from build123d import *
from build123d.topology import SkipClean

# Parameters (mm, degrees)
ESQUISSE1_R             = 2.1
ESQUISSE1_R_2           = 13.5
BOSS_EXTRU_1_DEPTH      = 3
ESQUISSE2_R             = 2.1
ENL_V_MAT_EXTRU_1_DEPTH = 3
ESQUISSE3_R             = 4.1
ESQUISSE3_R_2           = 2.1
BOSS_EXTRU_2_DEPTH      = 2
ENL_V_MAT_EXTRU_2_DEPTH = 3
CONG_1_R                = 20


with BuildPart() as part:
    # Esquisse1 → Boss.-Extru.1 (new body)
    with BuildSketch(Plane.XY):
        Polygon((22.273863607, -59.043416229), (-59.043416229, 22.273863607), (-22.273863607, 59.043416229), (59.043416229, -22.273863607), align=None)
        with Locations((0, 20)):
            Circle(ESQUISSE1_R, mode=Mode.SUBTRACT)
        Circle(ESQUISSE1_R_2, mode=Mode.SUBTRACT)
        with Locations((20, 0)):
            Circle(ESQUISSE1_R, mode=Mode.SUBTRACT)
        with Locations((0, -20)):
            Circle(ESQUISSE1_R, mode=Mode.SUBTRACT)
        with Locations((-20, 0)):
            Circle(ESQUISSE1_R, mode=Mode.SUBTRACT)
    extrude(amount=BOSS_EXTRU_1_DEPTH)

    # Esquisse2 → Enl_v. mat.-Extru.1 (cut)
    with BuildSketch(Plane.XY.offset(3)):
        with Locations((-37.123106012, 37.123106012)):
            Circle(ESQUISSE2_R)
        with Locations(Location((37.123106012, -37.123106012, 0), (0, 0, 180))):
            Circle(ESQUISSE2_R)
    extrude(amount=-ENL_V_MAT_EXTRU_1_DEPTH, mode=Mode.SUBTRACT)

    # Esquisse3 → Boss.-Extru.2 (add)
    # profile 1 of 6: a face of its own
    with SkipClean():  # the faces are left unmerged after this step: merging them gives an invalid solid
        with BuildSketch(Plane.XY.offset(3)):
            with Locations((37.123106012, -37.123106012)):
                Circle(ESQUISSE3_R)
            with Locations((37.123106012, -37.123106012)):
                Circle(ESQUISSE3_R_2, mode=Mode.SUBTRACT)
        # profile 2 of 6: a face of its own
        with BuildSketch(Plane.XY.offset(3)):
            with Locations((20, 0)):
                Circle(ESQUISSE3_R)
            with Locations((20, 0)):
                Circle(ESQUISSE3_R_2, mode=Mode.SUBTRACT)
        # profile 3 of 6: a face of its own
        with BuildSketch(Plane.XY.offset(3)):
            with Locations((0, -20)):
                Circle(ESQUISSE3_R)
            with Locations((0, -20)):
                Circle(ESQUISSE3_R_2, mode=Mode.SUBTRACT)
        # profile 4 of 6: a face of its own
        with BuildSketch(Plane.XY.offset(3)):
            with Locations((-20, 0)):
                Circle(ESQUISSE3_R)
            with Locations((-20, 0)):
                Circle(ESQUISSE3_R_2, mode=Mode.SUBTRACT)
        # profile 5 of 6: a face of its own
        with BuildSketch(Plane.XY.offset(3)):
            with Locations((-37.123106012, 37.123106012)):
                Circle(ESQUISSE3_R)
            with Locations((-37.123106012, 37.123106012)):
                Circle(ESQUISSE3_R_2, mode=Mode.SUBTRACT)
        # profile 6 of 6: a face of its own
        with BuildSketch(Plane.XY.offset(3)):
            with Locations((0, 20)):
                Circle(ESQUISSE3_R)
            with Locations((0, 20)):
                Circle(ESQUISSE3_R_2, mode=Mode.SUBTRACT)
        extrude(amount=BOSS_EXTRU_2_DEPTH)
    add(part.part.scale(1), mode=Mode.REPLACE)  # the faces are merged on a copy

    # Esquisse4 → Enl_v. mat.-Extru.2 (cut)
    with BuildSketch(Plane.XY.offset(3)):
        with BuildLine():
            Line((-35.355194284, 21.149212527), (-21.277194344, 35.355194284))
            ThreePointArc((-21.277194344, 35.355194284), (-7.135203496, 35.419185193), (-7.071212587, 21.277194344))
            Line((-7.071212587, 21.277194344), (-21.149212527, 7.071212587))
            ThreePointArc((-21.149212527, 7.071212587), (-35.291203375, 7.007221678), (-35.355194284, 21.149212527))
        make_face()
        with BuildLine():
            Line((21.149212527, -35.355194284), (35.355194284, -21.277194344))
            ThreePointArc((35.355194284, -21.277194344), (35.419185193, -7.135203496), (21.277194344, -7.071212587))
            Line((21.277194344, -7.071212587), (7.071212587, -21.149212527))
            ThreePointArc((7.071212587, -21.149212527), (7.007221678, -35.291203375), (21.149212527, -35.355194284))
        make_face()
    extrude(amount=-ENL_V_MAT_EXTRU_2_DEPTH, mode=Mode.SUBTRACT)

    # Cong_1
    cong_1_edges = [part.edges().sort_by_distance(p)[0] for p in [
        (22.273863607, -59.043416229, 1.5),
        (-59.043416229, 22.273863607, 1.5),
        (-22.273863607, 59.043416229, 1.5),
        (59.043416229, -22.273863607, 1.5),
    ]]
    fillet(cong_1_edges, radius=CONG_1_R)


solid = part.part
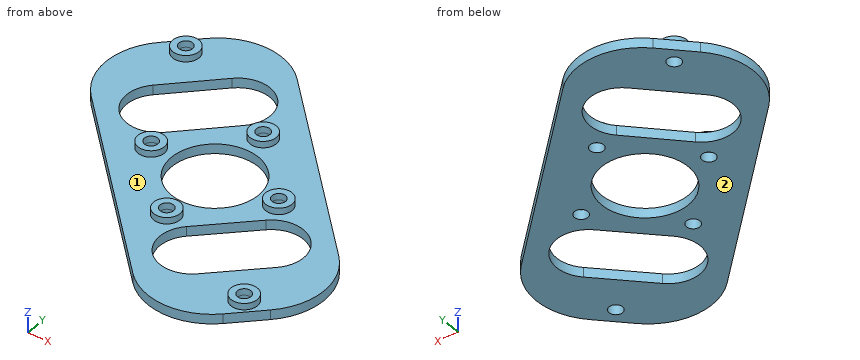
CAD build for the part. Positions are in the model's coordinates, mm. Face numbers are marked on the shaded views. A direction names the side the tool comes from. Round coordinates to 2 decimals unless told otherwise and drop trailing zeros. Write each loop counter-clockwise with the first axis right and the second up, starting at its lowest first coordinate (ties: lowest second). Pieces come first, ordered by that corner, then holes. Notation, with made-up numbers: M 68.5,17 L 78.5,17 A10 cw 78.5,33 Z; hole C -14,68.5 d11. An arc over 180 degrees is marked long. Use a Markdown table: item, result. Add a question column.
1. 3-axis set-ups, long thin cutter, end or side, ignore diameter. For the marked faces 1 and 2: which of +Z, -Z, +X, -X, +Y, -Y reach the whole face in a straight line?
2. Slice it at D-D on y = -25.5. Give the cut face in (x, z), then the cut area to 3 significant figures.
3. Slice it at A-A on y = 0. Give the cut face in (x, z).
4. Flat gauge pins, fed straight in: P1, Ø3, axis at x = -35, z = 0.5, coming from the -Y side; P2, Ø2, axis at x = 37.5, z = 2, coming from the +Y side. Where does each tip first touch, or does it go through?
5. Slice it at C-C on z = 2.25. Give the number of separate pieces and of enclosed holes in the cut face, then the cut area to 3 significant figures.
6. Drill centre lines: probe 1 along Y at (x, z) = (0, 3.45); probe 2 along X at (y, z) = (-12, 2); probe 3 along Y at (x, z) = (-18.5, 2.5). Where is each one in solid material? Low to high.
Reply:
| question | item | result |
|---|---|---|
| 1 | face 1 | +Z |
| 1 | face 2 | -Z, +X, -X, +Y, -Y |
| 2 | outline | M -11.27,0 L 4.5,0 L 4.5,3 L -11.27,3 Z; M 31.09,0 L 50.5,0 L 50.5,3 L 31.09,3 Z |
| 2 | area | 106 mm^2 |
| 3 | outline | M -36.77,0 L -22.1,0 L -22.1,5 L -24.1,5 L -24.1,3 L -36.77,3 Z; M -17.9,0 L -13.5,0 L -13.5,3 L -15.9,3 L -15.9,5 L -17.9,5 Z; M 13.5,0 L 17.9,0 L 17.9,5 L 15.9,5 L 15.9,3 L 13.5,3 Z; M 22.1,0 L 36.77,0 L 36.77,3 L 24.1,3 L 24.1,5 L 22.1,5 Z |
| 4 | P1 | stops at y = -3.27 |
| 4 | P2 | stops at y = 0.27 |
| 5 | separate pieces | 1 |
| 5 | enclosed holes | 9 |
| 5 | area | 3,550 mm^2 |
| 6 | probe 1 | y = -24.1 to -22.1, -17.9 to -15.9, 15.9 to 17.9, 22.1 to 24.1 |
| 6 | probe 2 | x = -24.77 to -6.18, 6.18 to 16.3, 38.08 to 47.92 |
| 6 | probe 3 | y = -18.27 to -1.47, 1.47 to 9.74, 37.33 to 50.4 |
